```python
from build123d import *

# Parameters (mm, degrees)
F1_DEPTH = 15
F3_START = -2
F2_R     = 4
F3_DEPTH = 40.5202370871
F4_D     = 1.75
F5_R     = 5


with BuildPart() as f1:
    # F0 (on Right) → F1 (new body, symmetric)
    with BuildSketch(Plane.YZ):
        Polygon((-5, 15.2480270107), (-5, -30), (0, -30), (0, 0), (8, 0), (26.3986550643, -1.9337765705), (26.3986550643, -16.9337765705), (23.3986550643, -16.9337765705), (23.3986550643, -21.9337765705), (31.3986550643, -21.9337765705), (31.3986550643, 2), align=None)
    extrude(amount=F1_DEPTH, both=True)

    # F2 (on face) → F3 (cut)
    with BuildSketch(Plane(origin=(0, 4.3157325251, 11.8573776612), x_dir=(1, 0, 0), z_dir=(0, 0.3420201433, 0.9396926208)).offset(F3_START)):
        with Locations((-6, -1.1789558201)):
            Circle(F2_R)
        with Locations((6, -1.1789558201)):
            Circle(F2_R)
    extrude(amount=-F3_DEPTH, mode=Mode.SUBTRACT)

    # F4 (through all)
    with Locations(Plane(origin=(0, 4.3157325251, 11.8573776612), x_dir=(1, 0, 0), z_dir=(0, 0.3420201433, 0.9396926208))):
        with Locations((6, -1.1789558201), (-6, -1.1789558201)):
            Hole(F4_D / 2)

    # F5
    f5_edges = [f1.edges().sort_by_distance(p)[0] for p in [
        (0, 31.398655, -21.933777),
    ]]
    fillet(f5_edges, radius=F5_R)


solid = f1.part
```
Here's how the part is built. I have some questions about the finished solid (model axes, mm). A direction names the side the tool comes from. Give positions to 0.01 mm unless a question says otherwise; leave off trailing zeros. Order: outer loops, then holes, each group sorted by start corner. A loop starts at its lowest first (then second) coordinate and runs counter-clockwise, first axis right, second up. Notation, with made-up numbers: (69, 46) - (75, 46) arc R26 cw to (75, 81) - close; hole circle Ø2 at (41, 62.25). An arc over 180 degrees is marked (long way). Answer as a JSON object with one key per item and string values. Group by question number.
Item 1: If we section it at C-C on x = 7.75: Please give me the cut outline in (y, z).
Item 2: Please list where these lines run through material, in increasing order: probe 1 along Y at (x, z) = (6, -8); probe 2 along Y at (x, z) = (-10, -26.5); probe 3 along Y at (x, z) = (-0.75, -3.5).
Item 3: If we section it at D-D on z = -8: Give the number of separate pieces and of enclosed holes in the cut face, and give its area (3 significant figures).
Item 4: If we section it at B-B on x = -6: Please give me the cut outline in (y, z).
Item 5: If we mould it in two halves opening along Z, with no side actions, what happens to faces 1 (the flat face through (0, 23.399, -19)), 2 (the flat face through (-5.167, 1.741, 10.666)), 3 (the flat face through (0.21, 13.454, 8.531))? For each: pulls with the +Z half, pulls with the -Z half, needs draft (parallel to the pull), parting line crosses it, or undercut.
Item 6: If we section it at A-A on x = 11: Please give me the cut outline in (y, z).
Item 7: Which directions (+Z, -Z, +X, -X, +Y, -Y) give clear straight access to the entire face, cutting with the end or side of a thin tool? Please do faces 4 (the flat face through (0, 25, -21.934)), 5 (the flat face through (0, 4, 0)), 6 (the flat face through (6.833, 1.741, 10.666)), 7 (the flat face through (0, 25, -16.934)).
Item 8: For P1, Ø3.5, axis at x = 3.5, y = 24.5, coming from the -Z side; P2, Ø12, axis at x = 2.5, y = 18.5, coming from the +Z side; P3, Ø1.5, axis at x = -2.5, y = 24.5, coming from the +Z side; P4, Ø12, axis at y = 26.5, z = 9.5, coming from the -X side, each with a flat end and sliding along its axis, tell me the tip position at first contact or that it passes through.
Result set:
{
 "1": {"outline": "(-5, -30) - (0, -30) - (0, -7.07) - (-5, -20.81) - close; (-5, 0.23) - (-0.86, 11.61) - (5.9, 9.15) - (2.57, 0) - (8, 0) - (26.4, -1.93) - (26.4, -16.93) - (23.4, -16.93) - (23.4, -21.93) - (26.4, -21.93) arc R5 ccw to (31.4, -16.93) - (31.4, 2) - (-5, 15.25) - close"},
 "2": {"probe 1": "26.4 to 31.4", "probe 2": "-5 to 0", "probe 3": "-5 to 0, 26.4 to 31.4"},
 "3": {"separate pieces": "4", "enclosed holes": "0", "area": "233 mm²"},
 "4": {"outline": "(-5, -30) - (0, -30) - (0, -8.25) - (-5, -21.99) - close; (-5, 1.4) - (-1.23, 11.75) - (1.7, 10.68) - (2.39, 12.56) - (-5, 15.25) - close; (3, 0) - (8, 0) - (26.4, -1.93) - (26.4, -16.93) - (23.4, -16.93) - (23.4, -21.93) - (26.4, -21.93) arc R5 ccw to (31.4, -16.93) - (31.4, 2) - (4.03, 11.96) - (3.35, 10.08) - (6.28, 9.01) - close"},
 "5": {"face 1": "needs draft", "face 2": "undercut", "face 3": "pulls with the +Z half"},
 "6": {"outline": "(-5, -30) - (0, -30) - (0, 0) - (8, 0) - (26.4, -1.93) - (26.4, -16.93) - (23.4, -16.93) - (23.4, -21.93) - (26.4, -21.93) arc R5 ccw to (31.4, -16.93) - (31.4, 2) - (-5, 15.25) - close"},
 "7": {"face 4": "-Z, +X, -X, +Y", "face 5": "-Z, +X, -X", "face 6": "none", "face 7": "+X, -X"},
 "8": {"P1": "z = -21.93", "P2": "z = 8.88", "P3": "z = 4.78", "P4": "x = -15"}
}
